Could you check a few things on this model? Use its own coordinates, in mm. A direction names the side the tool comes from. Round coordinates to 2 decimals unless told otherwise and drop trailing zeros. Loops run counter-clockwise (first coordinate to the right, second up) from the corner with the lowest first, then second, coordinate; pieces in that order, holes last. Notation, with made-up numbers: (18, 69) -> (58, 69) arc R13 cw to (58, 83) -> close; hole circle Ø4 at (-11, 32.25). An arc over 180 degrees is marked (long way). Write each question's results on one line, items separated by ' | '. Start each with the question number.
1) Imagine slicing it at B-B, the plane x = 25. List the corners of the cut face in (y, z) for me, plus the area to 3 significant figures.
2) If I drill on probe 1 along Z at (x, y) = (6.75, 23.5); probe 2 along Y at (x, z) = (18.5, -93.5); probe 3 along Y at (x, z) = (25, -98.6), over which ranges is the centre line in solid material (lowest first)?
3) Imagine slicing it at D-D, the plane x = 15. List the corners of the cut face in (y, z) for me.
4) For P1, Ø12, axis at x = 14, z = -37.5, coming from the -Y side; P2, Ø3, axis at x = 5, y = 5, coming from the +Z side, each with a flat end and sliding along its axis, tell me the tip position at first contact or that it passes through.
5) Which directions (+Z, -Z, +X, -X, +Y, -Y) give clear straight access to the entire face, cutting with the end or side of a thin tool? Please do faces 1 (the cylindrical face through (15, 39, -22.4)), 2 (the cylindrical face through (29.4, 0.57, 1.01)), 3 (the flat face through (19, 38, -48)).
6) We'd pull the mould along Y, two halves only. Please class faces 4 (the flat face through (19, 40, -48)), 5 (the cylindrical face through (4.65, 3.44, 0.99)), 6 (the cylindrical face through (23.73, 4.03, -98.99)), 7 (the flat face through (30, 39, -72)): pulls with the +Y half, pulls with the -Y half, needs draft (parallel to the pull), parting line crosses it, or undercut.
7) Imagine slicing it at A-A, the plane z = -44. List the corners of the cut face in (x, y) for me.
8) Imagine slicing it at C-C, the plane y = 5. List the corners of the cut face in (x, z) for me, plus the area to 3 significant figures.
from build123d import *

# Parameters (mm, degrees)
SKETCH_1_W          = 30
SKETCH_1_H          = 40
SKETCH_1_R          = 1.6
EXTRUDE_1_DEPTH     = 2
SKETCH_3_W          = 30
SKETCH_3_H          = 2
EXTRUDE_2_DEPTH     = 100
SKETCH_5_W          = 30
SKETCH_5_H          = 2
EXTRUDE_4_DEPTH     = 38
SKETCH_6_R          = 1.6
CUT_EXTRUDE_1_DEPTH = 114.595774569
CUT_EXTRUDE_2_DEPTH = 2
FILLET_1_R          = 2


with BuildPart() as part:
    # 草图1 → 凸台-拉伸1 (new body)
    with BuildSketch(Plane.XY):
        with Locations((15, 20)):
            Rectangle(SKETCH_1_W, SKETCH_1_H)
        with Locations((5, 5)):
            Circle(SKETCH_1_R, mode=Mode.SUBTRACT)
        with Locations((25, 5)):
            Circle(SKETCH_1_R, mode=Mode.SUBTRACT)
    extrude(amount=EXTRUDE_1_DEPTH)

    # 草图3 → 凸台-拉伸2 (add)
    with BuildSketch(Plane(origin=(0, 0, 0), x_dir=(-1, 0, 0), z_dir=(0, 0, -1))):
        with Locations((-15, 39)):
            Rectangle(SKETCH_3_W, SKETCH_3_H)
    extrude(amount=EXTRUDE_2_DEPTH)

    # 草图5 → 凸台-拉伸4 (add)
    with BuildSketch(Plane.XZ.offset(-38)):
        with Locations((15, -99)):
            Rectangle(SKETCH_5_W, SKETCH_5_H)
    extrude(amount=EXTRUDE_4_DEPTH)

    # 草图6 → 切除-拉伸1 (cut, through all)
    with BuildSketch(Plane.XY.offset(2)):
        with Locations((5, 5)):
            Circle(SKETCH_6_R)
        with Locations((25, 5)):
            Circle(SKETCH_6_R)
    extrude(amount=-CUT_EXTRUDE_1_DEPTH, mode=Mode.SUBTRACT)

    # 草图7 → 切除-拉伸2 (cut)
    with BuildSketch(Plane(origin=(0, 40, 0), x_dir=(1, 0, 0), z_dir=(0, 1, 0))):
        with BuildLine():
            Line((13.4, 24), (13.4, 74))
            ThreePointArc((13.4, 74), (15, 75.6), (16.6, 74))
            Line((16.6, 74), (16.6, 24))
            ThreePointArc((16.6, 24), (15, 22.4), (13.4, 24))
        make_face()
    extrude(amount=-CUT_EXTRUDE_2_DEPTH, mode=Mode.SUBTRACT)

    # 圆角1
    fillet_1_edges = [part.edges().sort_by_distance(p)[0] for p in [
        (0, 0, -99),
        (30, 0, -99),
        (30, 0, 1),
        (0, 0, 1),
    ]]
    fillet(fillet_1_edges, radius=FILLET_1_R)


solid = part.part
Checked values:
1) outline: (0, -100) -> (3.4, -100) -> (3.4, -98) -> (0, -98) -> close; (0, 0) -> (3.4, 0) -> (3.4, 2) -> (0, 2) -> close; (6.6, -100) -> (40, -100) -> (40, 2) -> (6.6, 2) -> (6.6, 0) -> (38, 0) -> (38, -98) -> (6.6, -98) -> close | area: 343 mm^2
2) probe 1: -100 to -98, 0 to 2 | probe 2: 38 to 40 | probe 3: 0 to 3.4, 6.6 to 40
3) outline: (0, -100) -> (40, -100) -> (40, -75.6) -> (38, -75.6) -> (38, -98) -> (0, -98) -> close; (0, 0) -> (38, 0) -> (38, -22.4) -> (40, -22.4) -> (40, 2) -> (0, 2) -> close
4) P1: y = 38 | P2: through
5) face 1: +Y, -Y | face 2: +Z, -Z, +X, -Y | face 3: +X, -X, -Y
6) face 4: pulls with the +Y half | face 5: undercut | face 6: undercut | face 7: needs draft
7) outline: (0, 38) -> (13.4, 38) -> (13.4, 40) -> (0, 40) -> close; (16.6, 38) -> (30, 38) -> (30, 40) -> (16.6, 40) -> close
8) outline: (0, -100) -> (3.4, -100) -> (3.4, -98) -> (0, -98) -> close; (0, 0) -> (3.4, 0) -> (3.4, 2) -> (0, 2) -> close; (6.6, -100) -> (23.4, -100) -> (23.4, -98) -> (6.6, -98) -> close; (6.6, 0) -> (23.4, 0) -> (23.4, 2) -> (6.6, 2) -> close; (26.6, -100) -> (30, -100) -> (30, -98) -> (26.6, -98) -> close; (26.6, 0) -> (30, 0) -> (30, 2) -> (26.6, 2) -> close | area: 94.4 mm^2
